For this review, use the dimensioned drawing (mm, ordinates from the lowest corner) and the shaded views. A direction names the side the tool comes from. Coordinates: 2 decimals unless noted, no trailing zeros. Order: outer loops, then holes, each group sorted by start corner. A loop starts at its lowest first (then second) coordinate and runs counter-clockwise, first axis right, second up. Notation, with made-up numbers: M 52,39 L 83,39 A22 cw 83,70 Z; hole C 32,-1 d6. An arc over 180 degrees is marked long. One line per item, written item: value.
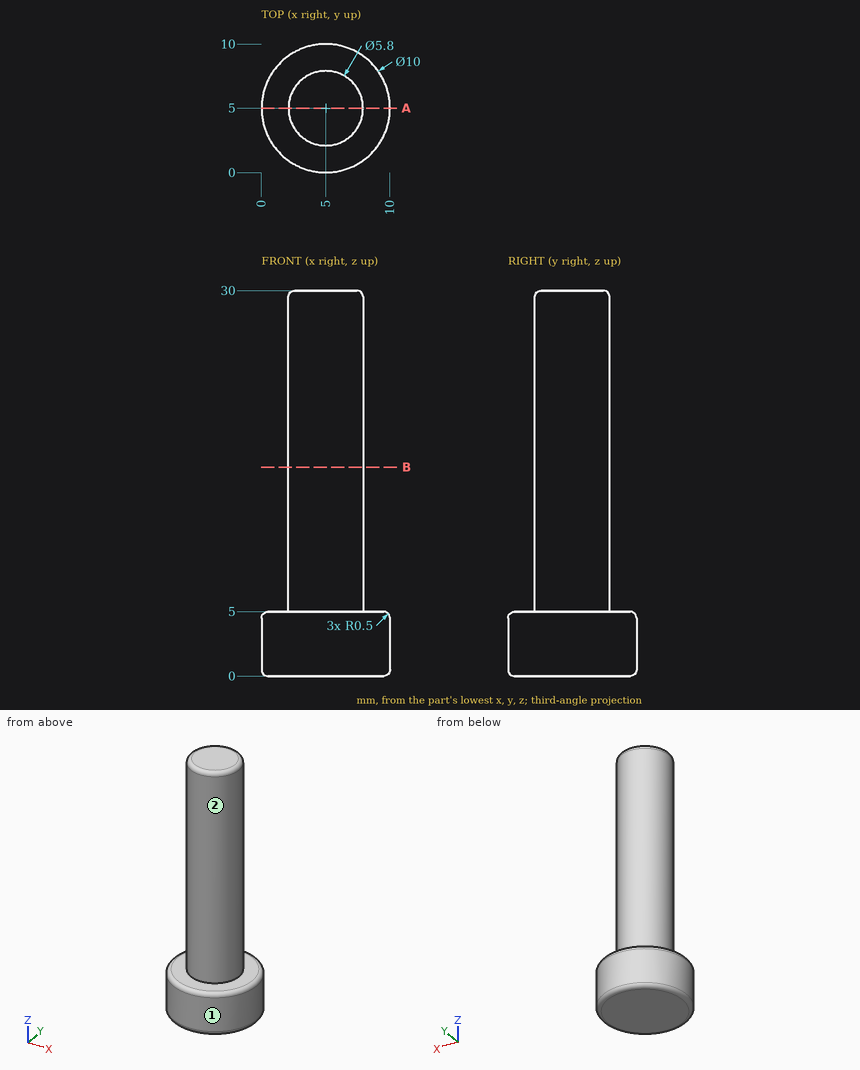
(1) Insertion check: pin 1 Ø1 at (y, z) = (2.5, 9.5) entering from -X; pin 2 Ø4 at (y, z) = (1.5, 25) entering from -X; pin 3 Ø1.5 at (x, z) = (4, 17) entering from -Y; pin 4 Ø1 at (y, z) = (8.5, 8) entering from -X. Each pin has a flat end and moves straight along its axis. Give the tip position at first contact, or say it passes through.
Geometry results:
pin 1: stops at x = 2.9
pin 2: stops at x = 2.52
pin 3: stops at y = 2.11
pin 4: passes through
(2) We need section A-A, the plane y = 5. State the section outline as (x, z) points, plus the area to 3 significant figures.
Geometry results:
outline: M 0,0.5 A0.5 ccw 0.5,0 L 9.5,0 A0.5 ccw 10,0.5 L 10,4.5 A0.5 ccw 9.5,5 L 7.9,5 L 7.9,29.5 A0.5 ccw 7.4,30 L 2.6,30 A0.5 ccw 2.1,29.5 L 2.1,5 L 0.5,5 A0.5 ccw 0,4.5 Z
area: 195 mm2
(3) We need section B-B, the plane z = 16.25. State the section outline as (x, y) points, plus the area to 3 significant figures.
Geometry results:
outline: C 5,5 d5.8
area: 26.4 mm2
(4) Tool access review of the marked faces 1 and 2: name each direction out of +Z, -Z, +X, -X, +Y, -Y from which nothing blocks a thin tool from reaching the whole face with its end or side.
Geometry results:
face 1: +Z, -Z
face 2: +Z
(5) For L1, parallel to Z at x = 4, y = 1.25; L2, parallel to Y at x = 5, z = 24.25; L3, parallel to Y at x = 5.75, z = 11.25, list the stretches that pass through material, from the lowest coordinate up.
Geometry results:
L1: z = 0 to 5
L2: y = 2.1 to 7.9
L3: y = 2.2 to 7.8
